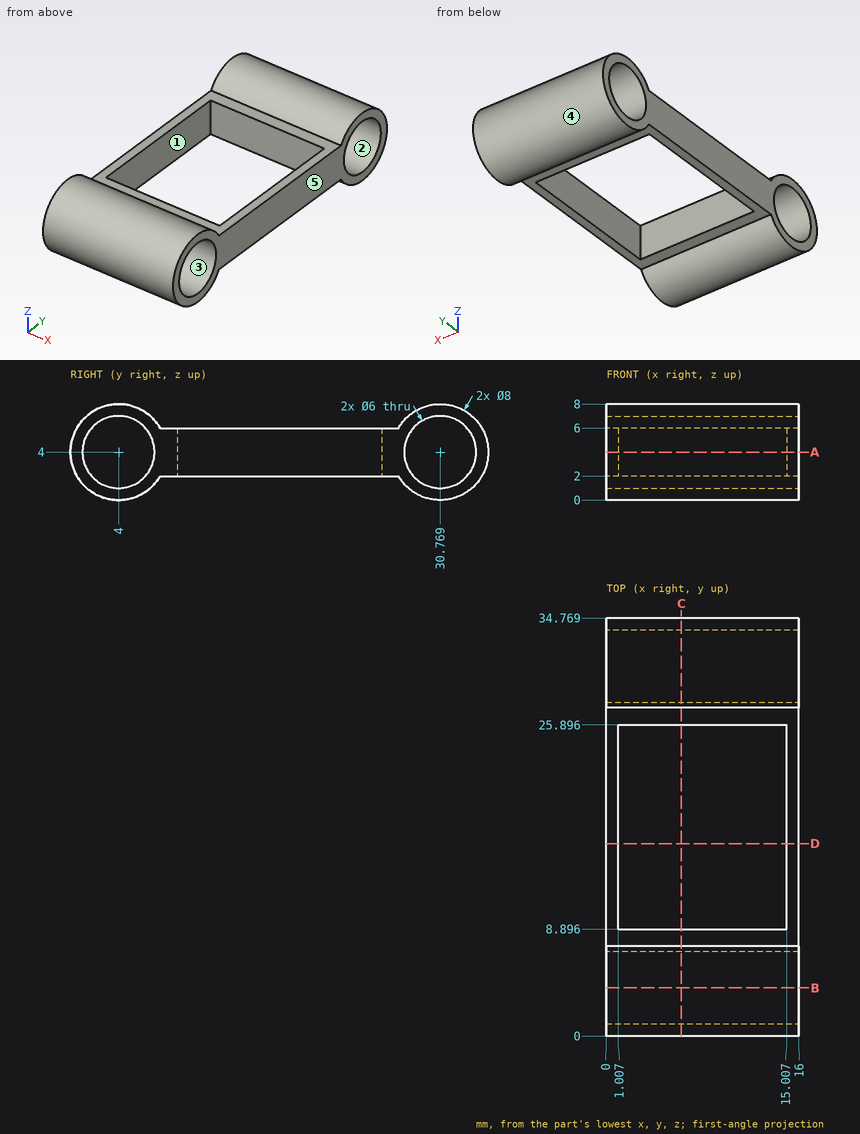
Design review of the part shown in the three views and the two pictorial views. Dimensions are in mm from the part's minimum x, y and z. A direction names the side the tool comes from. Round coordinates to 2 decimals unless told otherwise and drop trailing zeros. Loops run counter-clockwise (first coordinate to the right, second up) from the corner with the lowest first, then second, coordinate; pieces in that order, holes last. Notation, with made-up numbers: (63.5, 57.5) - (90.5, 57.5) arc R22 cw to (90.5, 70.5) - close; hole circle Ø2 at (-17, -10). An arc over 180 degrees is marked (long way). One line per item, written item: value. Start each with the question number.
Item 1: Clearance check with flat-ended pins moving along their axes: pin 1 Ø1 at (x, y) = (10, 23.5) entering from +Z; pin 2 Ø8 at (x, y) = (11.5, 5) entering from +Z; pin 3 Ø3 at (x, z) = (7, 6.5) entering from +Y; pin 4 Ø1 at (x, y) = (8.5, 8.5) entering from -Z. State where each tip first meets the part, or that it passes through.
Item 2: Take a section at B-B (y = 4). Give the boundary of the cut face in (x, z).
Item 3: For the marked faces 1 and 2, list the 3-axis set-ups (+Z, -Z, +X, -X, +Y, -Y) from which the entire face can be reached by the end or side of a thin tool; tool diameter is ignored.
Item 4: For L1, parallel to Z at x = 10.75, y = 4; L2, parallel to Y at x = 12.5, z = 5.75 (1 decimal); L3, parallel to Y at x = 6.25, z = 6.25 (1 decimal), list the stretches that pass through material, from the lowest coordinate up.
Item 5: The part is to be moulded in two halves that separate along Z. For the marked faces 3, 4 and 5, say which applies: +Z half, -Z half, draft (parallel to the pull), parting line (faces both ways), or undercut.
Item 6: Take a section at D-D (y = 16). Give the boundary of the cut face in (x, z).
Item 7: Take a section at C-C (x = 6.25). Give the boundary of the cut face in (y, z) (1 decimal).
Item 8: Take a section at A-A (z = 4). Give the boundary of the cut face in (x, y).
Answer below:
1. pin 1: passes through
1. pin 2: stops at z = 8
1. pin 3: stops at y = 34.64
1. pin 4: stops at z = 2
2. outline: (0, 0) - (16, 0) - (16, 1) - (0, 1) - close; (0, 7) - (16, 7) - (16, 8) - (0, 8) - close
3. face 1: +Z, -Z
3. face 2: +X, -X
4. L1: z = 0 to 1, 7 to 8
4. L2: y = 0.4 to 1.6, 6.4 to 8.9, 25.9 to 28.3, 33.2 to 34.4
4. L3: y = 0.7 to 2, 6 to 7.3, 27.5 to 28.8, 32.8 to 34.1
5. face 3: undercut
5. face 4: parting line
5. face 5: draft
6. outline: (0, 2) - (1.01, 2) - (1.01, 6) - (0, 6) - close; (15.01, 2) - (16, 2) - (16, 6) - (15.01, 6) - close
7. outline: (7.5, 2) - (8.9, 2) - (8.9, 6) - (7.5, 6) arc R4 ccw (long way) to start; (25.9, 2) - (27.3, 2) arc R4 ccw (long way) to (27.3, 6) - (25.9, 6) - close; hole circle Ø6 at (4, 4); hole circle Ø6 at (30.8, 4)
8. outline: (0, 0) - (16, 0) - (16, 1) - (0, 1) - close; (0, 7) - (16, 7) - (16, 27.77) - (0, 27.77) - close; (0, 33.77) - (16, 33.77) - (16, 34.77) - (0, 34.77) - close; hole (1.01, 8.9) - (15.01, 8.9) - (15.01, 25.9) - (1.01, 25.9) - close
